Design review of the part shown in the three views and the two pictorial views. Dimensions are in mm from the part's minimum x, y and z. A direction names the side the tool comes from. Give positions to 0.01 mm unless a question says otherwise; leave off trailing zeros. Write each loop counter-clockwise with the first axis right and the second up, starting at its lowest first coordinate (ties: lowest second). Pieces come first, ordered by that corner, then holes. Notation, with made-up numbers: (53.5, 17) -> (74.5, 17) arc R9 ccw to (74.5, 27) -> close; hole circle Ø4 at (24, 89). An arc over 180 degrees is marked (long way). Use CSV: the item, a comma, the result in double quotes.
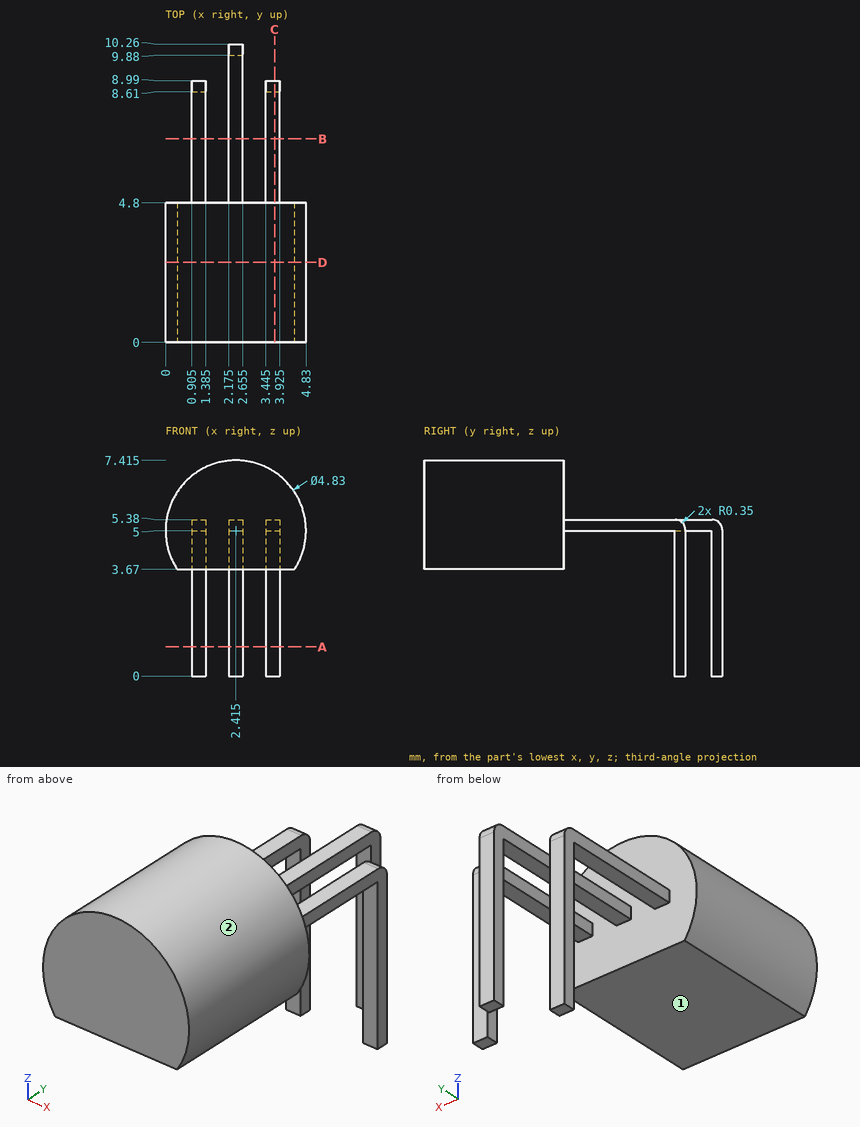
Q1. Insertion check: pin 1 (2 mm diameter, centred on x = 3.5, y = 6.5, fed in from +Z); pin 2 (1.1 mm diameter, centred on x = 3, z = 6.5, fed in from +Y); pin 3 (1 mm diameter, centred on y = 7.5, z = 2.5, fed in from -X). Each pin has a flat end and moves straight along its axis. Give the tip position at first contact, or say it passes through.
Derived:
pin 1,"stops at z = 5.38"
pin 2,"stops at y = 4.8"
pin 3,"passes through"
Q2. Machinability: for the marked faces 1 and 2, which of the approach directions +Z, -Z, +X, -X, +Y, -Y give a long, thin tool a straight path to every point of the face, cutting with its end or side? Answer none if there is none.
Derived:
face 1,"-Z, +X, -X, -Y"
face 2,"+Y, -Y"
Q3. Consider section A-A (z = 1). Write out the cut boundary in (x, y) (3 decimals).
Derived:
outline,"(0.905, 8.61) -> (1.385, 8.61) -> (1.385, 8.99) -> (0.905, 8.99) -> close; (2.175, 9.88) -> (2.655, 9.88) -> (2.655, 10.26) -> (2.175, 10.26) -> close; (3.445, 8.61) -> (3.925, 8.61) -> (3.925, 8.99) -> (3.445, 8.99) -> close"
Q4. Consider section B-B (y = 7). Write out the cut boundary in (x, z) (3 decimals).
Derived:
outline,"(0.905, 5) -> (1.385, 5) -> (1.385, 5.38) -> (0.905, 5.38) -> close; (2.175, 5) -> (2.655, 5) -> (2.655, 5.38) -> (2.175, 5.38) -> close; (3.445, 5) -> (3.925, 5) -> (3.925, 5.38) -> (3.445, 5.38) -> close"
Q5. To check wall thickness, follow probe 1 along X at (y, z) = (8, 5.25) (3 decimals); probe 2 along Y at (x, z) = (3.5, 6.75); probe 3 along Z at (x, y) = (1.2, 5). State the ranges of each line that lie inside material, in increasing order.
Derived:
probe 1,"x = 0.905 to 1.385, 2.175 to 2.655, 3.445 to 3.925"
probe 2,"y = 0 to 4.8"
probe 3,"z = 5 to 5.38"
Q6. Consider section C-C (x = 3.75). Write out the cut boundary in (y, z).
Derived:
outline,"(0, 3.67) -> (4.8, 3.67) -> (4.8, 5) -> (8.61, 5) -> (8.61, 0) -> (8.99, 0) -> (8.99, 5.03) arc R0.35 ccw to (8.64, 5.38) -> (4.8, 5.38) -> (4.8, 7.01) -> (0, 7.01) -> close"
Q7. Consider section D-D (y = 2.75). Write out the cut boundary in (x, z) (3 decimals), then the cut area to 3 significant figures.
Derived:
outline,"(0.399, 3.67) -> (4.431, 3.67) arc R2.415 ccw (long way) to start"
area,"15.2 mm2"
